```python
from build123d import *

# Parameters (mm, degrees)
SKETCH1_W           = 150
SKETCH1_H           = 125
BOSS_EXTRUDE1_DEPTH = 60
SHELL1_T            = -2.5


with BuildPart() as part:
    # Sketch1 → Boss-Extrude1 (new body)
    with BuildSketch(Plane(origin=(0, 0, 0), x_dir=(1, 0, 0), z_dir=(0, 1, 0))):
        Rectangle(SKETCH1_W, SKETCH1_H)
    extrude(amount=BOSS_EXTRUDE1_DEPTH)

    # Shell1
    shell1_openings = [part.faces().sort_by_distance(p)[0] for p in [
        (0, 60, 0),
        (0, 0, 0),
    ]]
    offset(amount=SHELL1_T, openings=shell1_openings, kind=Kind.INTERSECTION)


solid = part.part
```
The model under review builds one solid part; all positions refer to its coordinate system, in mm. A direction names the side the tool comes from. Round coordinates to 2 decimals unless told otherwise and drop trailing zeros. Loops run counter-clockwise (first coordinate to the right, second up) from the corner with the lowest first, then second, coordinate; pieces in that order, holes last.
1) The part is to be moulded in two halves that separate along X. For faces 3 (the face through (75, 30, 1)), 4 (the face through (-72.5, 30, 1)), 5 (the face through (-75, 30, 1)), 6 (the face through (-33.7, 60, -60.5)), say which applies: pulls with the +X half, pulls with the -X half, needs draft (parallel to the pull), parting line crosses it, or undercut.
Values follow:
face 3: pulls with the +X half
face 4: undercut
face 5: pulls with the -X half
face 6: needs draft
2) Tool access review of faces 1 (the face through (-1, 30, 62.5)), 2 (the face through (-1, 30, 60)): name each direction out of +Z, -Z, +X, -X, +Y, -Y from which nothing blocks a thin tool from reaching the whole face with its end or side.
Values follow:
face 1: +Z, +X, -X, +Y, -Y
face 2: +Y, -Y
3) Wall thickness on line 1 along Z through (x, y) = (13, 4.5); line 2 along X through (y, z) = (46.5, 3): over which ranges is each line inside the solid? List them lowest first.
Values follow:
line 1: z = -62.5 to -60, 60 to 62.5
line 2: x = -75 to -72.5, 72.5 to 75
4) Consider section B-B on z = -32.5. State the section outline as (x, y) points.
Values follow:
outline: (-75, 0) - (-72.5, 0) - (-72.5, 60) - (-75, 60) - close; (72.5, 0) - (75, 0) - (75, 60) - (72.5, 60) - close
5) Consider section C-C on y = 29.5. State the section outline as (x, z) points.
Values follow:
outline: (-75, -62.5) - (75, -62.5) - (75, 62.5) - (-75, 62.5) - close; hole (-72.5, -60) - (72.5, -60) - (72.5, 60) - (-72.5, 60) - close
6) Consider section A-A on x = -3.5. State the section outline as (y, z) points.
Values follow:
outline: (0, -62.5) - (60, -62.5) - (60, -60) - (0, -60) - close; (0, 60) - (60, 60) - (60, 62.5) - (0, 62.5) - close
